Source: CAD feature listing. Evaluate the final solid. Frame: model axes, mm. A direction names the side the tool comes from. Give positions to 0.01 mm unless a question says otherwise; leave off trailing zeros. Write each loop counter-clockwise with the first axis right and the second up, starting at its lowest first coordinate (ties: lowest second). Pieces come first, ordered by that corner, then holes. Notation, with made-up numbers: (81, 66.25) -> (123, 66.25) arc R23 cw to (123, 97.25) -> close; hole circle Ø2 at (5.25, 60). An arc over 180 degrees is marked (long way). Use one line per item in the form item = value. Start each with the question number.
(1) Cut plane B-B, the plane y = 44. Output: boundary loops of the cut face in (x, z), and give its area (3 significant figures).
(2) Cut plane A-A, the plane x = 0. Output: boundary loops of the cut face in (y, z).
(3) First-contact query: P1, Ø4, axis at x = 3, z = 11, coming from the +Y side; P2, Ø8, axis at x = -9, y = 50.5, coming from the -Z side; P3, Ø8, axis at x = 18, z = 20, coming from the +Y side. Flat tips, straight axial feed; report the tip coordinate or a pass-through.
(4) Draft query along Y for faces 4 (the face through (0, -6.251, 12)), 5 (the face through (-1.3, 45.1, 30.2)), 6 (the face through (5, 21, 25)), 7 (the face through (0, 6.251, 7)). Return one class per face: pulls with the +Y half, pulls with the -Y half, needs draft (parallel to the pull), parting line crosses it, or undercut.
(5) Cut plane D-D, the plane x = -13. Output: boundary loops of the cut face in (y, z), and give its area (3 significant figures).
(6) Material intervals for line 1 along Y through (x, z) = (0, 33); line 2 along Y through (x, z) = (-7.5, 20); line 3 along Z through (x, y) = (3, 26), sorted ascending. Write a range as from..to.
(7) Set-up query: faces 1 (the face through (0.58, 61.76, 20.07)), 2 (the face through (0, 22, 15)), 3 (the face through (-3.218, 21.056, 34.86)). Return all of +Z, -Z, +X, -X, +Y, -Y with unobstructed straight access to the full face (end or side cutting, diameter ignored); none if empty.
(8) Cut plane C-C, the plane z = 27.5. Output: boundary loops of the cut face in (x, y), and give its area (3 significant figures).
from build123d import *

# Parameters (mm, degrees)
F0_W     = 52.437798
F0_H     = 12.502962
F1_DEPTH = 15
F2_W     = 52.437798
F2_H     = 29.297988
F2_H_2   = 12.502962
F3_DEPTH = 10
F5_DEPTH = 10
F6_R     = 14.846163
F7_DEPTH = 20
F8_R     = 9.639432
F9_DEPTH = 45.001


with BuildPart() as f1:
    # F0 (on Top) → F1 (new body)
    with BuildSketch(Plane.XY):
        Rectangle(F0_W, F0_H)
    extrude(amount=F1_DEPTH)

    # F2 (on face) → F3 (join)
    with BuildSketch(Plane.XY.offset(15)):
        with Locations((0, 20.900475)):
            Rectangle(F2_W, F2_H)
        Rectangle(F2_W, F2_H_2)
    extrude(amount=F3_DEPTH)

    # F4 (on face) → F5 (join)
    with BuildSketch(Plane.XY.offset(25)):
        with BuildLine():
            Line((-26.218899, 35.549469), (26.218899, 35.549469))
            ThreePointArc((26.218899, 35.549469), (0, 61.768368), (-26.218899, 35.549469))
        make_face()
    extrude(amount=-F5_DEPTH)

    # F6 (on face) → F7 (join)
    with BuildSketch(Plane.XY.offset(25)):
        with Locations((0, 35.549469)):
            Circle(F6_R)
    extrude(amount=F7_DEPTH)

    # F8 (on face) → F9 (cut, through all)
    with BuildSketch(Plane.XY.offset(45)):
        with Locations((0, 35.549469)):
            Circle(F8_R)
    extrude(amount=-F9_DEPTH, mode=Mode.SUBTRACT)


solid = f1.part
Geometry says:
q1.outline = (-24.82, 15) -> (-4.64, 15) -> (-4.64, 45) -> (-12.21, 45) -> (-12.21, 25) -> (-24.82, 25) -> close; (4.64, 15) -> (24.82, 15) -> (24.82, 25) -> (12.21, 25) -> (12.21, 45) -> (4.64, 45) -> close
q1.area = 706 mm^2
q2.outline = (-6.25, 0) -> (6.25, 0) -> (6.25, 15) -> (25.91, 15) -> (25.91, 45) -> (20.7, 45) -> (20.7, 25) -> (-6.25, 25) -> close; (45.19, 15) -> (61.77, 15) -> (61.77, 25) -> (50.4, 25) -> (50.4, 45) -> (45.19, 45) -> close
q3.P1 = 6.25
q3.P2 = 15
q3.P3 = 57.72
q4.face_4 = pulls with the -Y half
q4.face_5 = undercut
q4.face_6 = needs draft
q4.face_7 = pulls with the +Y half
q5.outline = (-6.25, 0) -> (6.25, 0) -> (6.25, 15) -> (58.32, 15) -> (58.32, 25) -> (42.72, 25) -> (42.72, 45) -> (28.38, 45) -> (28.38, 25) -> (-6.25, 25) -> close
q5.area = 1,120 mm^2
q6.line_1 = 20.7..25.91, 45.19..50.4
q6.line_2 = -6.25..29.49, 41.6..60.67
q6.line_3 = 15..45
q7.face_1 = +Z, -Z, +Y
q7.face_2 = -Z, +X, -X, +Y
q7.face_3 = +Z
q8.outline = circle Ø29.69 at (0, 35.55); hole circle Ø19.28 at (0, 35.55)
q8.area = 401 mm^2
